Autodesk Inventor part; units mm, degrees
ref_plane "YZ Plane" through (0, 0, 0) normal (1, 0, 0) x (0, 1, 0)
ref_plane "XZ Plane" through (0, 0, 0) normal (0, 1, 0) x (-1, 0, 0)
ref_plane "XY Plane" through (0, 0, 0) normal (0, 0, 1) x (1, 0, 0)
sketch "Sketch1" plane through (0, 0, 0) normal (0, 0, 1) x (1, 0, 0)
  line L0 (-20, 3) -> (20, 3) construction
  line L1 (-20, -2) -> (20, -2)
  line L2 (20, 8) -> (-20, 8)
  arc A0 (-20, 8) -> (-20, -2) centre (-20, 3) ccw
  arc A1 (20, -2) -> (20, 8) centre (20, 3) ccw
  line L3 (-11, 16) -> (7.6141, 16)
  line L4 (7.6141, 16) -> (7.6141, 8)
  line L5 (7.6141, 8) -> (-11, 8)
  line L6 (-11, 8) -> (-11, 16)
  point P0 (0, 0)
  point P1 (0, 3)
  dimension "d0" = 10
  dimension "d2" = 40
extrude "Extrusion1" add sketch "Sketch1" along normal blind 5 contours A0 L2 A1 L1
extrude "Extrusion3" add sketch "Sketch1" along normal blind 5 contours L6 L3 L4 L2
properties material "Copper, Alloy"
Work out the finished part from the listing and answer in its coordinate system (mm). A direction names the side the tool comes from. Coordinates: 2 decimals unless noted, no trailing zeros. Loops run counter-clockwise (first coordinate to the right, second up) from the corner with the lowest first, then second, coordinate; pieces in that order, holes last.
1) Section C-C (x = 21) is taken. Give the vertices of the cut face in (y, z), plus the area to 3 significant figures.
Results:
outline: (-1.9, 0) - (7.9, 0) - (7.9, 5) - (-1.9, 5) - close
area: 49.0 mm2
2) Section A-A (z = 3.8) is taken. Give the vertices of the cut face in (x, y).
Results:
outline: (-20, -2) - (20, -2) arc R5 ccw to (20, 8) - (7.61, 8) - (7.61, 16) - (-11, 16) - (-11, 8) - (-20, 8) arc R5 ccw to start
3) For faces 1 (the flat face through (14, 8, 2)), 2 (the flat face through (-15, 8, 2)), 3 (the flat face through (0, 5, 5)), determine the directions among +Z, -Z, +X, -X, +Y, -Y from which every point of the face is accessible in a straight line to the end or side of a thin tool.
Results:
face 1: +Z, -Z, +X, +Y
face 2: +Z, -Z, -X, +Y
face 3: +Z, +X, -X, +Y, -Y
4) Section B-B (y = 14.25) is taken. Give the vertices of the cut face in (x, z).
Results:
outline: (-11, 0) - (7.61, 0) - (7.61, 5) - (-11, 5) - close
5) Consider probe 1 along X at (y, z) = (13.25, 4.35); probe 2 along Y at (x, z) = (15, 2.3); probe 3 along X at (y, z) = (1, 1.45). Determine where each line is inside the solid, lowest interval first.
Results:
probe 1: x = -11 to 7.61
probe 2: y = -2 to 8
probe 3: x = -24.58 to 24.58
6) Flat-ended cylindrical pins translate along their axes: pin 1 (2.5 mm diameter, centred on y = 14, z = 2.5, fed in from +X); pin 2 (2.5 mm diameter, centred on y = 11, z = 3.5, fed in from -X); pin 3 (1.5 mm diameter, centred on x = 12, z = 1.5, fed in from +Y). Find the tip coordinate at first contact, or state that the pin passes through.
Results:
pin 1: stops at x = 7.61
pin 2: stops at x = -11
pin 3: stops at y = 8
